Could you check a few things on this model? Use its own coordinates, in mm. Give positions to 0.01 mm unless a question says otherwise; leave off trailing zeros. Order: outer loops, then holes, each group sorted by start corner. A loop starts at its lowest first (then second) coordinate and runs counter-clockwise, first axis right, second up. Notation, with made-up numbers: (38.25, 8) -> (53.25, 8) arc R5 cw to (53.25, 12) -> close; hole circle Ø11 at (-21, 47.25). An arc over 180 degrees is marked (long way). Answer as CSV lines item,"result". Start each with the question number.
(1) I want a section at B-B (x = 0.75). Please give me the cut outline in (y, z), plus the area to 3 significant figures.
(2) I want a section at D-D (z = 0.35). Please give me the cut outline in (x, y), plus the area to 3 significant figures.
(3) I want a section at C-C (x = 0.3). Please give me the cut outline in (y, z).
(4) I want a section at A-A (y = 6.5). Please give me the cut outline in (x, z), plus the area to 3 significant figures.
(5) We'd pull the mould along Y, two halves only. Please class faces 1 (the face through (0.3, 6.787, 0.5)), 2 (the face through (0.3, 6.587, 0.4)), 3 (the face through (-0.45, 8, 1)), 4 (the face through (0, 0, 1)): released by +Y, released by -Y, zero draft, split by the parting line, or undercut.
(6) Will this pin go through, and if not, where does the flat tip stop? pin 1 Ø0.7 at (y, z) = (4, 1) entering from -X.
(7) I need wall thicknesses on L1, parallel to Z at x = 0.3, y = 0.1; L2, parallel to X at y = 8, z = 0.9; L3, parallel to Y at x = -0.15, z = 0.3. Which ranges of each line are inside material? Lowest first, please.
Autodesk Inventor part; units mm, degrees
ref_plane "YZ Plane" through (0, 0, 0) normal (1, 0, 0) x (0, 1, 0)
ref_plane "XZ Plane" through (0, 0, 0) normal (0, 1, 0) x (-1, 0, 0)
ref_plane "XY Plane" through (0, 0, 0) normal (0, 0, 1) x (1, 0, 0)
sketch "Boceto1" plane through (0, 0, 0) normal (0, 0, 1) x (1, 0, 0)
  line L0 (-0.3, 9.187) -> (-0.3, 6.787)
  line L1 (-0.3, 6.787) -> (0.9, 6.787)
  line L2 (0.9, 6.787) -> (0.9, 9.187)
  line L3 (0.9, 9.187) -> (1.05, 9.187)
  line L4 (1.05, 9.187) -> (1.05, 6.587)
  line L5 (0, 6.587) -> (-0.45, 6.587)
  line L6 (-0.45, 6.587) -> (-0.45, 9.187)
  line L7 (-0.45, 9.187) -> (-0.3, 9.187)
  line L8 (0.6, 0) -> (0.6, 6.587)
  line L9 (0.45, 6.587) -> (0.15, 6.587)
  line L10 (0, 6.587) -> (0, 0)
  line L11 (0, 0.3) -> (0.6, 0.3)
  line L12 (0.15, 0.3) -> (0.15, 6.587)
  line L13 (0.45, 0.3) -> (0.45, 6.587)
  line L14 (0.6, 6.587) -> (1.05, 6.587)
  line L15 (0, 0) -> (0.6, 0)
  point P0 (0, 0)
extrude "Extrusión1" add sketch "Boceto1" along normal blind 1.6 contours L0 L1 L2 L3 L4 L14 L8 L11 L13 L9 L12 L10 L5 L6 L7 | L11 L8 L15 L10
sketch "Boceto2" plane through (-0.3, 6.787, 0) normal (0, 1, 0) x (1, 0, 0)
  line L0 (1.2, 0) -> (0, 0)
  line L1 (0, 0) -> (0, -1.6)
  line L2 (1.2, -1.6) -> (0, -1.6)
  line L3 (1.2, 0) -> (1.2, -1.6)
  line L4 (0, -1.6) -> (0, -1.2)
  line L5 (0, -1.2) -> (0, -1)
  line L6 (0, -1) -> (1.2, -1)
  line L7 (1.2, 0) -> (1.2, -1.6)
  line L8 (0, -1.2) -> (1.2, -1.2)
  line L9 (1.2, -1.2) -> (1.2, -1)
  point P0 (0.3, 0)
  dimension "d2" = 0.4
  dimension "d3" = 0.2
  dimension "d4" = 1.2
extrude "Extrusión2" cut sketch "Boceto2" against normal blind 0.5 contours L3 L8 L1 L6
sketch "Boceto3" plane through (0.6, 0, 0) normal (1, 0, 0) x (0, 0, -1)
  line L0 (-1.6, 0.3) -> (0, 0.3)
  line L1 (-1, 6.587) -> (-1, 6.287)
  line L2 (-1, 6.287) -> (-1.2, 6.287)
  line L3 (-1.2, 6.287) -> (-1.2, 6.587)
  line L4 (-1.2, 6.587) -> (-1.6, 6.587)
  line L5 (-1.6, 0) -> (-1.6, 6.587)
  line L6 (0, 0) -> (-1.6, 0)
  line L7 (0, 0) -> (0, 6.587)
  line L8 (0, 6.587) -> (-1, 6.587)
  line L9 (-1.6, 0.3) -> (-1.6, 6.587)
  line L10 (-1.6, 0.3) -> (-1.2, 0.3)
  line L11 (-1.2, 0.3) -> (-1.2, 6.587)
  line L12 (-1.6, 6.587) -> (-1.2, 6.587)
  line L13 (-1.2, 6.587) -> (-1.2, 0.3)
  line L14 (-1.2, 0.3) -> (-1.6, 0.3)
  line L15 (-1.6, 0.3) -> (-1.6, 6.587)
  line L16 (0, 0.3) -> (0, 6.587)
  line L17 (0, 0.3) -> (-0.4, 0.3)
  line L18 (0, 0.3) -> (-1.6, 0.3)
  line L19 (0, 6.587) -> (-1.6, 6.587)
  line L20 (0, 6.587) -> (-0.4, 6.587)
  line L21 (-0.4, 6.587) -> (-0.4, 0.3)
  line L22 (-0.4, 0.3) -> (0, 0.3)
  line L23 (0, 0.3) -> (0, 6.587)
  point P0 (0, 0)
  dimension "d7" = 0.4
  dimension "d8" = 0.4
extrude "Extrusión3" cut sketch "Boceto3" against normal blind 0.9 contours L5 L4 L3 L11 L0 | L21 L8 L7 L0
sketch "Boceto4" plane through (0, 0.3, 0) normal (0, 1, 0) x (1, 0, 0)
  line L0 (0, 0) -> (0.6, 0)
  line L1 (0.6, 0) -> (0.6, -1.6)
  line L2 (0, -1.6) -> (0.6, -1.6)
  line L3 (0, 0) -> (0, -1.6)
  line L4 (0, -1.6) -> (0.6, -1.6)
  circle A0 centre (0.3, -1.35) radius 0.15
  line L5 (0, 0) -> (0, -1.6)
  circle A1 centre (0.3, -0.25) radius 0.15
  dimension "d12" = 0.3
extrude "Extrusión4" cut sketch "Boceto4" against normal blind 10 contours A0 | A1
sketch "Boceto5" plane through (0.6, 0, 0) normal (1, 0, 0) x (0, 0, -1)
  line L0 (-1.2, 0.3) -> (-1.6, 0.3)
  line L1 (-1.6, 0) -> (-1.6, 0.3)
  line L2 (0, 0) -> (-1.6, 0)
  line L3 (0, 0) -> (0, 0.3)
  line L4 (0, 0.3) -> (-0.4, 0.3)
  line L5 (-0.4, 0.3) -> (-0.4, 6.587)
  line L6 (-0.4, 6.587) -> (-1, 6.587)
  line L7 (-1, 6.587) -> (-1, 6.287)
  line L8 (-1, 6.287) -> (-1.2, 6.287)
  line L9 (-1.2, 6.287) -> (-1.2, 0.3)
  line L10 (-1.2, 6.287) -> (-1.2, 0.3)
  line L11 (-1.2, 6.287) -> (-1.1, 6.287)
  line L12 (-1, 6.287) -> (-1.2, 6.287)
  line L13 (-1.2, 0.3) -> (-1.1, 0.3)
  line L14 (-1.1, 0.3) -> (-1.1, 6.287)
  line L15 (-0.4, 0.3) -> (-0.5, 0.3)
  line L16 (-0.4, 0.3) -> (-1.2, 0.3)
  line L17 (-0.5, 0.3) -> (-0.5, 6.587)
  line L18 (-0.4, 0.3) -> (-0.4, 6.587)
  line L19 (-0.4, 6.587) -> (-0.4, 0.3)
  line L20 (-1.2, 0.3) -> (-1.2, 6.287)
  point P0 (0, 0)
  dimension "d15" = 0.1
  dimension "d16" = 0.1
  dimension "d17" = 0.1
extrude "Extrusión5" cut sketch "Boceto5" against normal blind 10 contours L9 L8 L14 L13 | L17 L6 L5 L15
sketch "Boceto6" plane through (0, 0, 0) normal (0, -1, 0) x (1, 0, 0)
  line L0 (0.9, 1.6) -> (0.9, 0)
  line L1 (0.9, 0) -> (-0.3, 0)
  line L2 (-0.3, 0) -> (-0.3, 1.6)
  line L3 (-0.3, 1.6) -> (0.9, 1.6)
  circle A0 centre (0.3, 1.25) radius 0.15
  circle A1 centre (0.3, 0.35) radius 0.15
  line L4 (0, 1.6) -> (0.6, 1.6)
  line L5 (0, 0) -> (0.6, 0)
extrude "Extrusión6" add sketch "Boceto6" against normal blind 0.3 contours L0 L1 L2 L3 | A0 | A1
sketch "Boceto7" plane through (0.9, 0, 0) normal (0, -1, 0) x (1, 0, 0)
  line L0 (0, 1.6) -> (0, 0)
  line L1 (0, 0) -> (-1.2, 0)
  line L2 (-1.2, 0) -> (-1.2, 1.6)
  line L3 (-1.2, 1.6) -> (0, 1.6)
  circle A0 centre (-0.6, 1.25) radius 0.15
  circle A1 centre (-0.6, 0.35) radius 0.15
  line L4 (-0.9, 1.6) -> (-0.3, 1.6)
  line L5 (-0.9, 0) -> (-0.3, 0)
  line L6 (-1.2, 0) -> (-1.2, 1.6)
  point P0 (-0.9, 0)
extrude "Extrusión7" cut sketch "Boceto7" against normal blind 0.5 contours A0 | A1
properties part number "learnbotAgarreServo"
Final values:
1,outline,"(0, 0) -> (0.3, 0) -> (0.3, 1.6) -> (0, 1.6) -> close; (6.59, 0) -> (6.79, 0) -> (6.79, 1) -> (6.59, 1) -> close; (6.59, 1.2) -> (6.79, 1.2) -> (6.79, 1.6) -> (6.59, 1.6) -> close"
1,area,"0.760 mm²"
2,outline,"(-0.45, 6.59) -> (1.05, 6.59) -> (1.05, 9.19) -> (0.9, 9.19) -> (0.9, 6.79) -> (-0.3, 6.79) -> (-0.3, 9.19) -> (-0.45, 9.19) -> close; (-0.3, 0) -> (0.15, 0) -> (0.15, 0.3) -> (-0.3, 0.3) -> close; (0.45, 0) -> (0.9, 0) -> (0.9, 0.3) -> (0.45, 0.3) -> close"
2,area,"1.29 mm²"
3,outline,"(0, 0) -> (0.3, 0) -> (0.3, 0.2) -> (0, 0.2) -> close; (0, 0.5) -> (0.3, 0.5) -> (0.3, 1.1) -> (0, 1.1) -> close; (0, 1.4) -> (0.3, 1.4) -> (0.3, 1.6) -> (0, 1.6) -> close; (6.59, 0) -> (6.79, 0) -> (6.79, 1) -> (6.59, 1) -> close; (6.59, 1.2) -> (6.79, 1.2) -> (6.79, 1.6) -> (6.59, 1.6) -> close"
4,outline,"(0, 0.5) -> (0.15, 0.5) -> (0.15, 1) -> (0, 1) -> close; (0.45, 0.5) -> (0.6, 0.5) -> (0.6, 1) -> (0.45, 1) -> close"
4,area,"0.150 mm²"
5,face 1,"released by +Y"
5,face 2,"undercut"
5,face 3,"zero draft"
5,face 4,"released by -Y"
6,pin 1,"x = 0"
7,L1,"0 to 0.2, 0.5 to 1.1, 1.4 to 1.6"
7,L2,"-0.45 to -0.3, 0.9 to 1.05"
7,L3,"0 to 0.3, 6.59 to 6.79"
